The listing builds one solid part. Answer for the finished solid, in the listing's coordinates (mm). A direction names the side the tool comes from. Coordinates: 2 decimals unless noted, no trailing zeros. Write each loop counter-clockwise with the first axis right and the second up, starting at its lowest first coordinate (ties: lowest second). Pieces come first, ordered by that corner, then holes.
(1) The part is cut by section B-B on z = -26. Determine the outline of the cut face in (x, y).
(2) Which of the six approach directions +Z, -Z, +X, -X, +Y, -Y give full straight-line access (tool end or side, diameter ignored) to faces 1 (the cylindrical face through (1.65, 15.42, -47.67)), 2 (the flat face through (0, 48, -44.45))?
(3) For a pull along Y with two mould halves and no side action, classify faces 3 (the flat face through (-34, 96.393, 0)), 4 (the flat face through (-34, 0, 0)), 5 (the cylindrical face through (34.881, 80.463, -1.852)), 6 (the flat face through (0, 48, 44.45)) as +Y half, -Y half, draft (parallel to the pull), parting line (faces both ways), or undercut.
(4) The part is cut by section C-C on y = 12.5. Determine the outline of the cut face in (x, z).
(5) The part is cut by section D-D on x = 27.5. Determine the outline of the cut face in (y, z).
(6) The part is cut by section A-A on x = 0. Determine the outline of the cut face in (y, z), plus the area to 3 significant figures.
(7) Straight lines are drawn through the part: line 1 (X direction, y = 82.5, z = -30); line 2 (Z direction, x = -6.5, y = 83). For each, find the intervals that lie inside material, in ascending order.
from build123d import *

# Parameters (mm, degrees)
SKETCH2_W           = 76.2
SKETCH2_H           = 101.6
SKETCH2_W_2         = 63.5
SKETCH2_H_2         = 88.9
EXTRUDE_THIN1_DEPTH = 96.393
SKETCH3_R           = 7.62
CUT_EXTRUDE1_DEPTH  = 102.6
SKETCH4_R           = 14.224
CUT_EXTRUDE2_DEPTH  = 77.2


with BuildPart() as part:
    # Sketch2 → Extrude-Thin1 (new body)
    with BuildSketch(Plane(origin=(0, 0, 0), x_dir=(1, 0, 0), z_dir=(0, 1, 0))):
        Rectangle(SKETCH2_W, SKETCH2_H)
        Rectangle(SKETCH2_W_2, SKETCH2_H_2, mode=Mode.SUBTRACT)
    extrude(amount=EXTRUDE_THIN1_DEPTH)

    # Sketch3 → Cut-Extrude1 (cut, through all)
    with BuildSketch(Plane(origin=(0, 0, -50.8), x_dir=(-1, 0, 0), z_dir=(0, 0, -1))):
        with Locations((0, 22.86)):
            Circle(SKETCH3_R)
    extrude(amount=-CUT_EXTRUDE1_DEPTH, mode=Mode.SUBTRACT)

    # Sketch4 → Cut-Extrude2 (cut, through all)
    with BuildSketch(Plane.ZY.offset(38.1)):
        with Locations((0, 66.360000122)):
            Circle(SKETCH4_R)
    extrude(amount=-CUT_EXTRUDE2_DEPTH, mode=Mode.SUBTRACT)


solid = part.part
Model answer:
1. outline: (-38.1, 0) - (-31.75, 0) - (-31.75, 96.39) - (-38.1, 96.39) - close; (31.75, 0) - (38.1, 0) - (38.1, 96.39) - (31.75, 96.39) - close
2. face 1: +Z, -Z
2. face 2: +Y, -Y
3. face 3: +Y half
3. face 4: -Y half
3. face 5: undercut
3. face 6: draft
4. outline: (-38.1, -50.8) - (38.1, -50.8) - (38.1, 50.8) - (-38.1, 50.8) - close; hole (-31.75, -44.45) - (31.75, -44.45) - (31.75, 44.45) - (-31.75, 44.45) - close
5. outline: (0, -50.8) - (96.39, -50.8) - (96.39, -44.45) - (0, -44.45) - close; (0, 44.45) - (96.39, 44.45) - (96.39, 50.8) - (0, 50.8) - close
6. outline: (0, -50.8) - (15.24, -50.8) - (15.24, -44.45) - (0, -44.45) - close; (0, 44.45) - (15.24, 44.45) - (15.24, 50.8) - (0, 50.8) - close; (30.48, -50.8) - (96.39, -50.8) - (96.39, -44.45) - (30.48, -44.45) - close; (30.48, 44.45) - (96.39, 44.45) - (96.39, 50.8) - (30.48, 50.8) - close
6. area: 1,030 mm2
7. line 1: x = -38.1 to -31.75, 31.75 to 38.1
7. line 2: z = -50.8 to -44.45, 44.45 to 50.8
